Build history of the part. All positions in model axes, mm. A direction names the side the tool comes from. Round coordinates to 2 decimals unless told otherwise and drop trailing zeros. Loops run counter-clockwise (first coordinate to the right, second up) from the corner with the lowest first, then second, coordinate; pieces in that order, holes last.
from build123d import *

# Parameters (mm, degrees)
CROQUIS1_W                   = 200
CROQUIS1_H                   = 120
SALIENTE_EXTRUIR1_DEPTH      = 40
CROQUIS2_W                   = 193.6
CROQUIS2_H                   = 113.6
CORTAR_EXTRUIR1_DEPTH        = 36
CROQUIS3_W                   = 71.5
CROQUIS3_H                   = 25.4
CORTAR_EXTRUIR2_DEPTH        = 3.5
CROQUIS4_R                   = 3.75
SALIENTE_EXTRUIR2_DEPTH      = 12.2
CROQUIS5_W                   = 71.5
CROQUIS5_H                   = 4
SALIENTE_EXTRUIR3_DEPTH      = 5
CROQUIS6_W                   = 7.5
CROQUIS6_H                   = 113.6
SALIENTE_EXTRUIR4_DEPTH      = 2
SALIENTE_EXTRUIR4_DEPTH_BACK = 5
CROQUIS7_R                   = 4.5
CORTAR_EXTRUIR3_DEPTH        = 3.3
CROQUIS6_5_R                 = 5
SALIENTE_EXTRUIR5_DEPTH      = 36
CROQUIS6_6_R                 = 5
SALIENTE_EXTRUIR6_DEPTH      = 5
SALIENTE_EXTRUIR6_DEPTH_BACK = 5
CROQUIS8_R                   = 2.5
CORTAR_EXTRUIR4_DEPTH        = 20
CROQUIS9_R                   = 2.5
CORTAR_EXTRUIR5_DEPTH        = 11


with BuildPart() as part:
    # Croquis1 → Saliente-Extruir1 (new body)
    with BuildSketch(Plane(origin=(0, 0, 0), x_dir=(1, 0, 0), z_dir=(0, 1, 0))):
        Rectangle(CROQUIS1_W, CROQUIS1_H)
    extrude(amount=SALIENTE_EXTRUIR1_DEPTH)

    # Croquis2 → Cortar-Extruir1 (cut)
    with BuildSketch(Plane(origin=(0, 40, 0), x_dir=(1, 0, 0), z_dir=(0, 1, 0))):
        Rectangle(CROQUIS2_W, CROQUIS2_H)
    extrude(amount=-CORTAR_EXTRUIR1_DEPTH, mode=Mode.SUBTRACT)

    # Croquis3 → Cortar-Extruir2 (cut)
    with BuildSketch(Plane.XY.offset(60)):
        with Locations((0, 20.3)):
            Rectangle(CROQUIS3_W, CROQUIS3_H)
    extrude(amount=-CORTAR_EXTRUIR2_DEPTH, mode=Mode.SUBTRACT)

    # Croquis4 → Saliente-Extruir2 (add)
    with BuildSketch(Plane.XY.offset(60)):
        with Locations((-37.5, 35.8)):
            Circle(CROQUIS4_R)
        with Locations((37.5, 35.8)):
            Circle(CROQUIS4_R)
        with Locations((37.5, 4.8)):
            Circle(CROQUIS4_R)
        with Locations((-37.5, 4.8)):
            Circle(CROQUIS4_R)
    extrude(amount=-SALIENTE_EXTRUIR2_DEPTH)

    # Croquis5 → Saliente-Extruir3 (add)
    with BuildSketch(Plane.XY.offset(60)):
        with Locations((0, 5.6)):
            Rectangle(CROQUIS5_W, CROQUIS5_H)
        with Locations((0, 35)):
            Rectangle(CROQUIS5_W, CROQUIS5_H)
    extrude(amount=-SALIENTE_EXTRUIR3_DEPTH)

    # Croquis6 → Saliente-Extruir4 (add, two sides)
    with BuildSketch(Plane(origin=(0, 4, 0), x_dir=(1, 0, 0), z_dir=(0, 1, 0))) as saliente_extruir4_sk:
        with Locations((-78.05, 0)):
            Rectangle(CROQUIS6_W, CROQUIS6_H)
        with Locations((-46.83, 0)):
            Rectangle(CROQUIS6_W, CROQUIS6_H)
        with Locations((-15.61, 0)):
            Rectangle(CROQUIS6_W, CROQUIS6_H)
        with Locations((15.61, 0)):
            Rectangle(CROQUIS6_W, CROQUIS6_H)
        with Locations((46.83, 0)):
            Rectangle(CROQUIS6_W, CROQUIS6_H)
        with Locations((78.05, 0)):
            Rectangle(CROQUIS6_W, CROQUIS6_H)
    extrude(amount=SALIENTE_EXTRUIR4_DEPTH)
    extrude(saliente_extruir4_sk.sketch, amount=-SALIENTE_EXTRUIR4_DEPTH_BACK)

    # Croquis7 → Cortar-Extruir3 (cut)
    with BuildSketch(Plane(origin=(0, 0, -60), x_dir=(-1, 0, 0), z_dir=(0, 0, -1))):
        with Locations((0, 20)):
            Circle(CROQUIS7_R)
    extrude(amount=-CORTAR_EXTRUIR3_DEPTH, mode=Mode.SUBTRACT)

    # Croquis6_5 → Saliente-Extruir5 (add)
    with BuildSketch(Plane(origin=(0, 4, 0), x_dir=(1, 0, 0), z_dir=(0, 1, 0))):
        with Locations((-90, 50)):
            Circle(CROQUIS6_5_R)
        with Locations((90, -50)):
            Circle(CROQUIS6_5_R)
    extrude(amount=SALIENTE_EXTRUIR5_DEPTH)

    # Croquis6_6 → Saliente-Extruir6 (add, two sides)
    with BuildSketch(Plane(origin=(0, 4, 0), x_dir=(1, 0, 0), z_dir=(0, 1, 0))) as saliente_extruir6_sk:
        with Locations((90, 50)):
            Circle(CROQUIS6_6_R)
        with Locations((-90, -50)):
            Circle(CROQUIS6_6_R)
    extrude(amount=SALIENTE_EXTRUIR6_DEPTH)
    extrude(saliente_extruir6_sk.sketch, amount=-SALIENTE_EXTRUIR6_DEPTH_BACK)

    # Croquis8 → Cortar-Extruir4 (cut)
    with BuildSketch(Plane(origin=(0, 40, 0), x_dir=(1, 0, 0), z_dir=(0, 1, 0))):
        with Locations((-90, 50)):
            Circle(CROQUIS8_R)
        with Locations((90, -50)):
            Circle(CROQUIS8_R)
    extrude(amount=-CORTAR_EXTRUIR4_DEPTH, mode=Mode.SUBTRACT)

    # Croquis9 → Cortar-Extruir5 (cut, through all)
    with BuildSketch(Plane(origin=(0, 9, 0), x_dir=(1, 0, 0), z_dir=(0, 1, 0))):
        with Locations((-90, -50)):
            Circle(CROQUIS9_R)
        with Locations((90, 50)):
            Circle(CROQUIS9_R)
    extrude(amount=-CORTAR_EXTRUIR5_DEPTH, mode=Mode.SUBTRACT)


solid = part.part
(1) Slice it at A-A on y = 22.5. List the corners of the cut face in (x, z).
Responses:
outline: (-100, -60) - (-3.74, -60) - (-3.74, -56.8) - (-96.8, -56.8) - (-96.8, 56.8) - (-35.75, 56.8) - (-35.75, 60) - (-100, 60) - close; circle Ø10 at (-90, -50); (3.74, -60) - (100, -60) - (100, 60) - (35.75, 60) - (35.75, 56.8) - (96.8, 56.8) - (96.8, -56.8) - (3.74, -56.8) - close; circle Ø10 at (90, 50); hole circle Ø5 at (-90, -50); hole circle Ø5 at (90, 50)
(2) Probe line 1 (X direction, y = 23.5, z = 11.5); line 2 (Z direction, x = -37.5, y = 4.5); line 3 (Y direction, x = 0, z = -58). List the from-to ranges inside material, lowest first.
Responses:
line 1: x = -100 to -96.8, 96.8 to 100
line 2: z = -60 to -56.8, 47.8 to 60
line 3: y = 0 to 15.5, 24.5 to 40
(3) Pull direction X, two halves, no side cores. Call faces 1 (the face through (100, 20, 1)), 2 (the face through (93, 6, -54)), 3 (the face through (-88, 40, -48)): +X half, -X half, draft (parallel to the pull), parting line (faces both ways), or undercut.
Responses:
face 1: +X half
face 2: undercut
face 3: draft
(4) Pin check, flat tips, straight feed: P1, Ø0.5, axis at x = -15.5, y = -0.5, coming from the +Z side; P2, Ø6, axis at x = 62, z = -37, coming from the -Y side; P3, Ø7.5, axis at x = 87.5, z = 24.5, coming from the +Y side; P4, Ø4.5, axis at x = 90, z = -50, coming from the +Y side. Stop position of each tip, or through.
Responses:
P1: stops at z = 56.8
P2: stops at y = 0
P3: stops at y = 4
P4: passes through
(5) Slice it at C-C on x = 0. List the corners of the cut face in (y, z), plus the area to 3 significant figures.
Responses:
outline: (0, -60) - (15.5, -60) - (15.5, -56.8) - (4, -56.8) - (4, 55) - (7.6, 55) - (7.6, 60) - (0, 60) - close; (24.5, -60) - (40, -60) - (40, -56.8) - (24.5, -56.8) - close; (33, 55) - (37, 55) - (37, 56.8) - (40, 56.8) - (40, 60) - (33, 60) - close
area: 614 mm2
(6) Which spindle directions (+Z, -Z, +X, -X, +Y, -Y) get a long thin tool onto all of the face, cutting with end or side? Do faces 4 (the face through (92, -1, -48)), 5 (the face through (-89, 4, -1)), 6 (the face through (41.077, 36.926, 52.63)), 7 (the face through (92.688, -0.493, -54.216)). Say none if no direction does.
Responses:
face 4: +Z, -Z, +X, -X, -Y
face 5: +Y
face 6: none
face 7: -Y
(7) Slice it at B-B on x = 90. List the corners of the cut face in (y, z).
Responses:
outline: (-1, -55) - (0, -55) - (0, -60) - (40, -60) - (40, -56.8) - (4, -56.8) - (4, -55) - (9, -55) - (9, -52.5) - (-1, -52.5) - close; (-1, -47.5) - (9, -47.5) - (9, -45) - (4, -45) - (4, 45) - (40, 45) - (40, 47.5) - (20, 47.5) - (20, 52.5) - (40, 52.5) - (40, 55) - (4, 55) - (4, 56.8) - (40, 56.8) - (40, 60) - (0, 60) - (0, -45) - (-1, -45) - close
(8) Slice it at D-D on z = 50. Count the separate pieces of the cut face and the enclosed holes in it, plus the area to 3 significant figures.
Responses:
separate pieces: 4
enclosed holes: 0
area: 1,580 mm2
